The model under review builds one solid part; all positions refer to its coordinate system, in mm. Give positions to 0.01 mm unless a question says otherwise; leave off trailing zeros. Write each loop counter-clockwise with the first axis right and the second up, starting at its lowest first coordinate (ties: lowest second). Pieces come first, ordered by that corner, then holes. Notation, with made-up numbers: (-36, 35.5) -> (-30, 35.5) arc R6 ccw to (-30, 45.5) -> close; hole circle Ø7 at (9, 54). An arc over 180 degrees is marked (long way). Use CSV: the item, a comma, the result in double quotes.
```python
from build123d import *

# Parameters (mm, degrees)
F0_W     = 50
F0_H     = 50
F1_DEPTH = 3.5
F2_R     = 1.75
F3_DEPTH = 3.501


with BuildPart() as f1:
    # F0 (on Top) → F1 (new body)
    with BuildSketch(Plane.XY):
        with Locations((25, -25)):
            Rectangle(F0_W, F0_H)
    extrude(amount=F1_DEPTH)

    # F2 (on face) → F3 (cut, through all)
    with BuildSketch(Plane.XY.offset(3.5)):
        with Locations((4, -4)):
            Circle(F2_R)
        with Locations((14, -4)):
            Circle(F2_R)
        with Locations((24, -4)):
            Circle(F2_R)
        with Locations((34, -4)):
            Circle(F2_R)
        with Locations((44, -4)):
            Circle(F2_R)
        with Locations((44, -14)):
            Circle(F2_R)
        with Locations((34, -14)):
            Circle(F2_R)
        with Locations((24, -14)):
            Circle(F2_R)
        with Locations((14, -14)):
            Circle(F2_R)
        with Locations((4, -14)):
            Circle(F2_R)
        with Locations((4, -24)):
            Circle(F2_R)
        with Locations((14, -24)):
            Circle(F2_R)
        with Locations((24, -24)):
            Circle(F2_R)
        with Locations((34, -24)):
            Circle(F2_R)
        with Locations((44, -24)):
            Circle(F2_R)
        with Locations((4, -34)):
            Circle(F2_R)
        with Locations((14, -34)):
            Circle(F2_R)
        with Locations((24, -34)):
            Circle(F2_R)
        with Locations((34, -34)):
            Circle(F2_R)
        with Locations((44, -34)):
            Circle(F2_R)
        with Locations((4, -44)):
            Circle(F2_R)
        with Locations((14, -44)):
            Circle(F2_R)
        with Locations((24, -44)):
            Circle(F2_R)
        with Locations((34, -44)):
            Circle(F2_R)
        with Locations((44, -44)):
            Circle(F2_R)
    extrude(amount=-F3_DEPTH, mode=Mode.SUBTRACT)


solid = f1.part
```
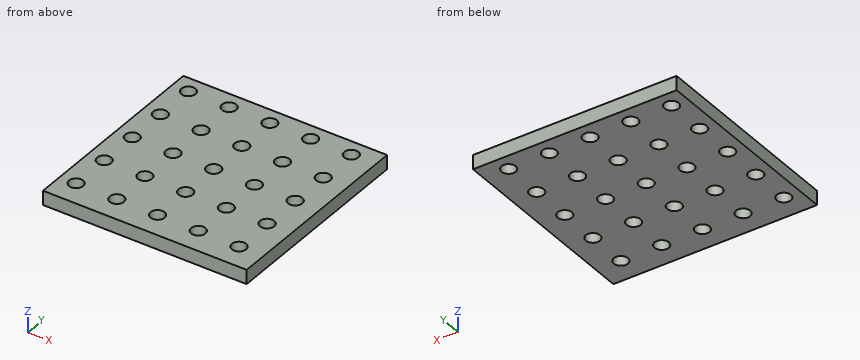
Q1. To check wall thickness, follow probe 1 along Y at (x, z) = (34, 2.25); probe 2 along X at (y, z) = (-25, 2.1); probe 3 along X at (y, z) = (-4.5, 2.8). State the ranges of each line that lie inside material, in increasing order.
Derived:
probe 1,"y = -50 to -45.75, -42.25 to -35.75, -32.25 to -25.75, -22.25 to -15.75, -12.25 to -5.75, -2.25 to 0"
probe 2,"x = 0 to 2.56, 5.44 to 12.56, 15.44 to 22.56, 25.44 to 32.56, 35.44 to 42.56, 45.44 to 50"
probe 3,"x = 0 to 2.32, 5.68 to 12.32, 15.68 to 22.32, 25.68 to 32.32, 35.68 to 42.32, 45.68 to 50"
Q2. Consider section C-C (x = 44). Write out the cut boundary in (y, z).
Derived:
outline,"(-50, 0) -> (-45.75, 0) -> (-45.75, 3.5) -> (-50, 3.5) -> close; (-42.25, 0) -> (-35.75, 0) -> (-35.75, 3.5) -> (-42.25, 3.5) -> close; (-32.25, 0) -> (-25.75, 0) -> (-25.75, 3.5) -> (-32.25, 3.5) -> close; (-22.25, 0) -> (-15.75, 0) -> (-15.75, 3.5) -> (-22.25, 3.5) -> close; (-12.25, 0) -> (-5.75, 0) -> (-5.75, 3.5) -> (-12.25, 3.5) -> close; (-2.25, 0) -> (0, 0) -> (0, 3.5) -> (-2.25, 3.5) -> close"
Q3. Consider section A-A (z = 2.6). State how many separate pieces and enclosed holes the cut face has, then the cut area to 3 significant figures.
Derived:
separate pieces,"1"
enclosed holes,"25"
area,"2,260 mm2"
Q4. Consider section B-B (y = -14). Write out the cut boundary in (x, z).
Derived:
outline,"(0, 0) -> (2.25, 0) -> (2.25, 3.5) -> (0, 3.5) -> close; (5.75, 0) -> (12.25, 0) -> (12.25, 3.5) -> (5.75, 3.5) -> close; (15.75, 0) -> (22.25, 0) -> (22.25, 3.5) -> (15.75, 3.5) -> close; (25.75, 0) -> (32.25, 0) -> (32.25, 3.5) -> (25.75, 3.5) -> close; (35.75, 0) -> (42.25, 0) -> (42.25, 3.5) -> (35.75, 3.5) -> close; (45.75, 0) -> (50, 0) -> (50, 3.5) -> (45.75, 3.5) -> close"
